Can you work these out from the model? Positions are in its coordinate system, mm. Face numbers are marked on the shaded views. Give positions to 0.01 mm unless a question says otherwise; leave off trailing zeros.
Item 1: I'm going to push flat-ended pins straight in: pin 1 Ø1.5 at (y, z) = (0.5, 9.5) entering from +X; pin 2 Ø2 at (y, z) = (2, 10) entering from -X. Where does each tip first touch, or does it pass through?
Item 2: If we mould it in two halves opening along X, with no side actions, what happens to the marked faces 1, 2 and 3? For each: +X half, -X half, draft (parallel to the pull), parting line (faces both ways), or undercut.
Item 3: If I drill on line 1 along X through (y, z) = (0.8, -4); line 2 along X through (y, z) = (1.4, 6); line 3 along Y through (x, z) = (-0.25, 7.5), over which ranges is the centre line in solid material (lowest first)?
```python
from build123d import *

# Parameters (mm, degrees)
F1_ANGLE = 180


with BuildPart() as f1:
    # F0 (on Front) → F1 (revolve)
    with BuildSketch(Plane.XZ):
        with BuildLine():
            Line((2.921, -1.016), (2.921, 0))
            Line((2.921, 0), (3.556, 0))
            ThreePointArc((3.556, 0), (2.503044, 9.11053), (0, 17.933524))
            Line((0, 17.933524), (0, 6.971839))
            Line((0, 6.971839), (1.5875, 6.12775))
            Line((1.5875, 6.12775), (1.5875, -1.016))
            Line((1.5875, -1.016), (1.5875, -5.08))
            Line((1.5875, -5.08), (2.921, -5.08))
            Line((2.921, -5.08), (2.921, -1.016))
        make_face()
    revolve(axis=Axis((0, 0, 12.452682), (0, 0, 1)), revolution_arc=F1_ANGLE)


solid = f1.part
```
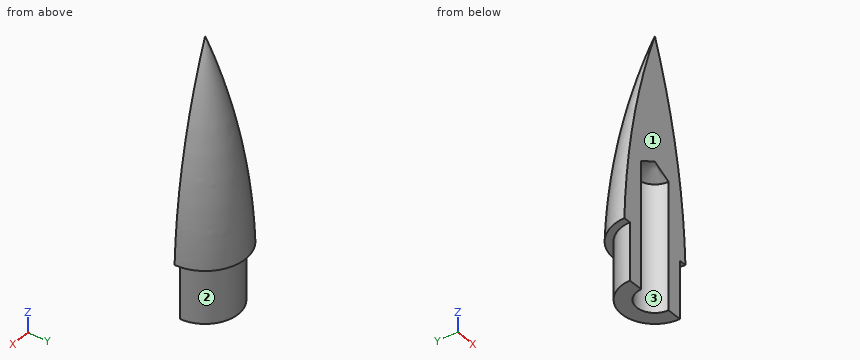
Results list:
1. pin 1: stops at x = 2.55
1. pin 2: stops at x = -2.15
2. face 1: draft
2. face 2: parting line
2. face 3: undercut
3. line 1: x = -2.81 to -1.37, 1.37 to 2.81
3. line 2: x = -2.69 to -0.75, 0.75 to 2.69
3. line 3: y = 0 to 2.79
